from build123d import *

# Parameters (mm, degrees)
SKETCH1_W           = 7.5
SKETCH1_H           = 28
SKETCH1_R           = 1.4
BOSS_EXTRUDE1_DEPTH = 250.2
CUT_EXTRUDE1_DEPTH  = 2


with BuildPart() as part:
    # Sketch1 → Boss-Extrude1 (new body)
    with BuildSketch(Plane(origin=(0, 0, 0), x_dir=(1, 0, 0), z_dir=(0, 1, 0))):
        Rectangle(SKETCH1_W, SKETCH1_H)
        with Locations(Location((1.25, -9, 0), (0, 0, 270))):
            Circle(SKETCH1_R, mode=Mode.SUBTRACT)
        with Locations(Location((1.25, 9, 0), (0, 0, 270))):
            Circle(SKETCH1_R, mode=Mode.SUBTRACT)
    extrude(amount=BOSS_EXTRUDE1_DEPTH)

    # Sketch3 → Cut-Extrude1 (cut)
    with BuildSketch(Plane.ZY.offset(3.75)):
        with BuildLine():
            Line((-1.476181201, 137.36625), (-3.572358506, 125.744325))
            ThreePointArc((-3.572358506, 125.744325), (-3.63, 125.1), (-3.572358506, 124.455675))
            Line((-3.572358506, 124.455675), (-1.476181201, 112.83375))
            ThreePointArc((-1.476181201, 112.83375), (0, 111.6), (1.476181201, 112.83375))
            Line((1.476181201, 112.83375), (3.572358506, 124.455675))
            ThreePointArc((3.572358506, 124.455675), (3.63, 125.1), (3.572358506, 125.744325))
            Line((3.572358506, 125.744325), (1.476181201, 137.36625))
            ThreePointArc((1.476181201, 137.36625), (0, 138.6), (-1.476181201, 137.36625))
        make_face()
    extrude(amount=-CUT_EXTRUDE1_DEPTH, mode=Mode.SUBTRACT)


solid = part.part
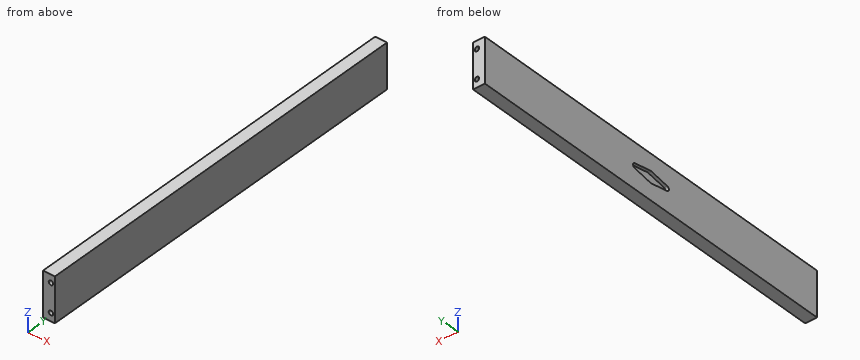
Geometry: final body of the model. Coordinates: model frame, mm. Round coordinates to 2 decimals unless told otherwise and drop trailing zeros. Write each loop counter-clockwise with the first axis right and the second up, starting at its lowest first coordinate (ties: lowest second). Pieces come first, ordered by that corner, then holes. Notation, with made-up numbers: M -35,43 L -26,43 A27 ccw -26,79 Z; hole C 52,46 d7. An arc over 180 degrees is marked long. Write item = value, one per line.
Item 1: Section query A-A on x = 1.25. Return loops of the section in (y, z).
Findings:
outline = M 0,-14 L 250.2,-14 L 250.2,-10.4 L 0,-10.4 Z; M 0,-7.6 L 250.2,-7.6 L 250.2,7.6 L 0,7.6 Z; M 0,10.4 L 250.2,10.4 L 250.2,14 L 0,14 Z
Item 2: Material intervals for line 1 along Z through (x, y) = (1.5, 144); line 2 along X through (y, z) = (116.5, 9); line 3 along Z through (x, y) = (0.25, 129), sorted ascending. Write a range as [from, to].
Findings:
line_1 = [-14, -10.38], [-7.62, 7.62], [10.38, 14]
line_2 = [-3.75, -0.15], [2.65, 3.75]
line_3 = [-14, -9.98], [-8.02, 8.02], [9.98, 14]
Item 3: Pin query (flat end, axial travel): P1, Ø2, axis at x = 1.25, z = -9, coming from the +Y side. Return the tip coordinate at first contact, or that it passes through.
Findings:
P1 = through
Item 4: Section query B-B on y = 177. Return loops of the section in (x, z), then the cut area to 3 significant figures.
Findings:
outline = M -3.75,-14 L 3.75,-14 L 3.75,14 L -3.75,14 Z; hole C 1.25,-9 d2.8; hole C 1.25,9 d2.8
area = 198 mm^2
